Can you work these out from the model? Positions are in its coordinate system, mm. Face numbers are marked on the shaded views. Give positions to 0.01 mm unless a question says otherwise; leave off trailing zeros. Order: outer loops, then holes, each group sorted by start corner. A loop starts at its lowest first (then second) coordinate and runs counter-clockwise, first axis right, second up. Notation, with made-up numbers: (82.5, 61) - (89.5, 61) arc R20 cw to (89.5, 90) - close; hole circle Ø10 at (-37.75, 13.25). An arc over 180 degrees is marked (long way). Answer as CSV lines item,"result".
Autodesk Inventor part; units mm, degrees
ref_plane "YZ Plane" through (0, 0, 0) normal (1, 0, 0) x (0, 1, 0)
ref_plane "XZ Plane" through (0, 0, 0) normal (0, 1, 0) x (-1, 0, 0)
ref_plane "XY Plane" through (0, 0, 0) normal (0, 0, 1) x (1, 0, 0)
sketch "Sketch1" plane through (0, 0, 0) normal (0, 0, 1) x (1, 0, 0)
  circle A0 centre (0, 0) radius 11.75
  circle A1 centre (0, 0) radius 36.75
  dimension "d0" = 23.5
  dimension "d1" = 73.5
extrude "Extrusion1" add sketch "Sketch1" along normal blind 12.7
sketch "Sketch2" plane through (0, 0, 12.7) normal (0, 0, 1) x (1, 0, 0)
  circle A0 centre (15, 0) radius 1
  circle A1 centre (0, 30) radius 1
  circle A2 centre (12.1353, 8.8168) radius 1
  circle A3 centre (4.6353, 14.2658) radius 1
  circle A4 centre (-4.6353, 14.2658) radius 1
  circle A5 centre (-12.1353, 8.8168) radius 1
  circle A6 centre (-15, 0) radius 1
  circle A7 centre (-12.1353, -8.8168) radius 1
  circle A8 centre (-4.6353, -14.2658) radius 1
  circle A9 centre (4.6353, -14.2658) radius 1
  circle A10 centre (12.1353, -8.8168) radius 1
  circle A11 centre (-17.6336, 24.2705) radius 1
  circle A12 centre (-28.5317, 9.2705) radius 1
  circle A13 centre (-28.5317, -9.2705) radius 1
  circle A14 centre (-17.6336, -24.2705) radius 1
  circle A15 centre (0, -30) radius 1
  circle A16 centre (17.6336, -24.2705) radius 1
  circle A17 centre (28.5317, -9.2705) radius 1
  circle A18 centre (28.5317, 9.2705) radius 1
  circle A19 centre (17.6336, 24.2705) radius 1
  point P0 (0, 0)
  dimension "d4" = 2
  dimension "d5" = 2
  dimension "d6" = 15
  dimension "d7" = 30
  dimension "d10" = 360
  dimension "d14" = 360
extrude "Extrusion2" cut sketch "Sketch2" against normal through all
sketch "Sketch3" plane through (0, 0, 12.7) normal (0, 0, 1) x (1, 0, 0)
  line L0 (-1, 18) -> (1, 18)
  line L1 (1, 18) -> (1, 26)
  line L2 (1, 26) -> (-1, 26)
  line L3 (-1, 26) -> (-1, 18)
  line L4 (-11.3892, 13.9745) -> (-9.7711, 15.1501)
  line L5 (-9.7711, 15.1501) -> (-14.4734, 21.6222)
  line L6 (-14.4734, 21.6222) -> (-16.0914, 20.4467)
  line L7 (-16.0914, 20.4467) -> (-11.3892, 13.9745)
  line L8 (-17.428, 4.6112) -> (-16.81, 6.5134)
  line L9 (-16.81, 6.5134) -> (-24.4185, 8.9855)
  line L10 (-24.4185, 8.9855) -> (-25.0365, 7.0834)
  line L11 (-25.0365, 7.0834) -> (-17.428, 4.6112)
  line L12 (-16.81, -6.5134) -> (-17.428, -4.6112)
  line L13 (-17.428, -4.6112) -> (-25.0365, -7.0834)
  line L14 (-25.0365, -7.0834) -> (-24.4185, -8.9855)
  line L15 (-24.4185, -8.9855) -> (-16.81, -6.5134)
  line L16 (-9.7711, -15.1501) -> (-11.3892, -13.9745)
  line L17 (-11.3892, -13.9745) -> (-16.0914, -20.4467)
  line L18 (-16.0914, -20.4467) -> (-14.4734, -21.6222)
  line L19 (-14.4734, -21.6222) -> (-9.7711, -15.1501)
  line L20 (1, -18) -> (-1, -18)
  line L21 (-1, -18) -> (-1, -26)
  line L22 (-1, -26) -> (1, -26)
  line L23 (1, -26) -> (1, -18)
  line L24 (11.3892, -13.9745) -> (9.7711, -15.1501)
  line L25 (9.7711, -15.1501) -> (14.4734, -21.6222)
  line L26 (14.4734, -21.6222) -> (16.0914, -20.4467)
  line L27 (16.0914, -20.4467) -> (11.3892, -13.9745)
  line L28 (17.428, -4.6112) -> (16.81, -6.5134)
  line L29 (16.81, -6.5134) -> (24.4185, -8.9855)
  line L30 (24.4185, -8.9855) -> (25.0365, -7.0834)
  line L31 (25.0365, -7.0834) -> (17.428, -4.6112)
  line L32 (16.81, 6.5134) -> (17.428, 4.6112)
  line L33 (17.428, 4.6112) -> (25.0365, 7.0834)
  line L34 (25.0365, 7.0834) -> (24.4185, 8.9855)
  line L35 (24.4185, 8.9855) -> (16.81, 6.5134)
  line L36 (9.7711, 15.1501) -> (11.3892, 13.9745)
  line L37 (11.3892, 13.9745) -> (16.0914, 20.4467)
  line L38 (16.0914, 20.4467) -> (14.4734, 21.6222)
  line L39 (14.4734, 21.6222) -> (9.7711, 15.1501)
  point P0 (0, 0)
  point P1 (0, 18)
  point P2 (-10.5801, 14.5623)
  point P3 (-17.119, 5.5623)
  point P4 (-17.119, -5.5623)
  point P5 (-10.5801, -14.5623)
  point P6 (0, -18)
  point P7 (10.5801, -14.5623)
  point P8 (17.119, -5.5623)
  point P9 (17.119, 5.5623)
  point P10 (10.5801, 14.5623)
  dimension "d18" = 18
  dimension "d19" = 26
  dimension "d20" = 2
  dimension "d23" = 360
extrude "Extrusion3" cut sketch "Sketch3" against normal through all
properties part number "SG03" material "Rubber"
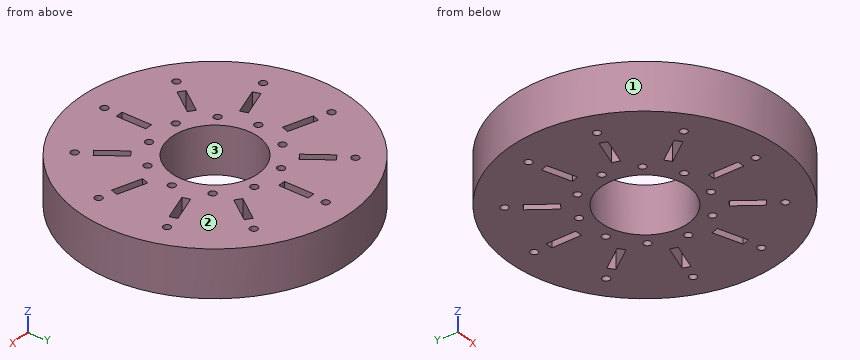
1) I want a section at B-B on x = 7.5. Write out the boundary of the cut face in (y, z), plus the area to 3 significant figures.
Answer block:
outline,"(-35.98, 0) - (-9.05, 0) - (-9.05, 12.7) - (-35.98, 12.7) - close; (9.05, 0) - (35.98, 0) - (35.98, 12.7) - (9.05, 12.7) - close"
area,"684 mm2"
2) I want a section at A-A on y = 0. Write out the boundary of the cut face in (x, z).
Answer block:
outline,"(-36.75, 0) - (-16, 0) - (-16, 12.7) - (-36.75, 12.7) - close; (-14, 0) - (-11.75, 0) - (-11.75, 12.7) - (-14, 12.7) - close; (11.75, 0) - (14, 0) - (14, 12.7) - (11.75, 12.7) - close; (16, 0) - (36.75, 0) - (36.75, 12.7) - (16, 12.7) - close"
3) I need wall thicknesses on line 1 along Y through (x, z) = (0, 10.5); line 2 along X through (y, z) = (-15, 5); line 3 along Y through (x, z) = (-21.5, 9.5). Which ranges of each line are inside material? Lowest first, please. Write a range as [from, to].
Answer block:
line 1,"[-36.75, -31], [-29, -26], [-18, -11.75], [11.75, 18], [26, 29], [31, 36.75]"
line 2,"[-33.55, -12.13], [-9.98, -5.31], [-3.96, 3.96], [5.31, 9.98], [12.13, 33.55]"
line 3,"[-29.8, -8.04], [-5.93, 5.93], [8.04, 29.8]"
4) I want a section at D-D on y = -17. Write out the boundary of the cut face in (x, z), plus the area to 3 significant figures.
Answer block:
outline,"(-32.58, 0) - (-13.59, 0) - (-13.59, 12.7) - (-32.58, 12.7) - close; (-11.12, 0) - (11.12, 0) - (11.12, 12.7) - (-11.12, 12.7) - close; (13.59, 0) - (32.58, 0) - (32.58, 12.7) - (13.59, 12.7) - close"
area,"765 mm2"
5) I'm going to push flat-ended pins straight in: P1, Ø0.6, axis at x = 0, z = 5.5, coming from the -Y side; P2, Ø5, axis at x = 3, z = 6.5, coming from the +Y side; P3, Ø3, axis at y = 5.5, z = 11, coming from the -X side. Where does each tip first touch, or does it pass through?
Answer block:
P1,"y = -36.75"
P2,"y = 36.75"
P3,"x = -36.53"
6) I want a section at C-C on y = 30. Write out the boundary of the cut face in (x, z), plus the area to 3 significant figures.
Answer block:
outline,"(-21.23, 0) - (-1, 0) - (-1, 12.7) - (-21.23, 12.7) - close; (1, 0) - (21.23, 0) - (21.23, 12.7) - (1, 12.7) - close"
area,"514 mm2"
7) If we mould it in two halves opening along X, with no side actions, what happens to the marked faces 1, 2 and 3? For each: +X half, -X half, draft (parallel to the pull), parting line (faces both ways), or undercut.
Answer block:
face 1,"parting line"
face 2,"draft"
face 3,"undercut"
